Read the model definition and answer for the solid it produces. Units are mm, in the model's axes. A direction names the side the tool comes from. Coordinates: 2 decimals unless noted, no trailing zeros. Write each loop counter-clockwise with the first axis right and the second up, starting at its lowest first coordinate (ties: lowest second). Pieces come first, ordered by that corner, then holes.
from build123d import *

# Parameters (mm, degrees)
PAD002_DEPTH    = 2
FILLET003_R     = 0.4
POCKET010_DEPTH = 0.1


with BuildPart() as part:
    # Sketch009 → Pad002 (new body)
    with BuildSketch(Plane.XY):
        Polygon((-1.675, -0.66), (1.675, -0.66), (1.675, -1.66), (0.5, -1.66), (0.5, -20.32), (1.5, -20.32), (1.5, -21.82), (-1.5, -21.82), (-1.5, -20.32), (-0.5, -20.32), (-0.5, -1.66), (-1.675, -1.66), align=None)
    extrude(amount=PAD002_DEPTH)

    # Fillet003
    fillet003_edges = [part.edges().sort_by_distance(p)[0] for p in [
        (-1.675, -1.66, 1),
        (-1.675, -0.66, 1),
        (1.675, -0.66, 1),
        (1.675, -1.66, 1),
        (0.5, -1.66, 1),
        (-0.5, -1.66, 1),
        (-0.5, -20.32, 1),
        (-1.5, -20.32, 1),
        (-1.5, -21.82, 1),
        (1.5, -21.82, 1),
        (1.5, -20.32, 1),
        (0.5, -20.32, 1),
    ]]
    fillet(fillet003_edges, radius=FILLET003_R)

    # Fillet003 Face5 → Pocket010 (cut)
    with BuildSketch(Plane(origin=(0, -11.4600006044, 2), x_dir=(0, 1, 0), z_dir=(0, 0, 1))):
        with BuildLine():
            Line((9.8000006044, 1.275), (9.8000006044, 0.9))
            ThreePointArc((9.8000006044, 0.9), (9.6828433168, 0.6171572875), (9.4000006044, 0.5))
            Line((9.4000006044, 0.5), (-8.4599993956, 0.5))
            ThreePointArc((-8.4599993956, 0.5), (-8.7428421081, 0.6171572875), (-8.8599993956, 0.9))
            Line((-8.8599993956, 0.9), (-8.8599993956, 1.1))
            ThreePointArc((-8.8599993956, 1.1), (-8.9771566832, 1.3828427125), (-9.2599993956, 1.5))
            Line((-9.2599993956, 1.5), (-9.9599993956, 1.5))
            ThreePointArc((-9.9599993956, 1.5), (-10.2428421081, 1.3828427125), (-10.3599993956, 1.1))
            Line((-10.3599993956, 1.1), (-10.3599993956, -1.1))
            ThreePointArc((-10.3599993956, -1.1), (-10.2428421081, -1.3828427125), (-9.9599993956, -1.5))
            Line((-9.9599993956, -1.5), (-9.2599993956, -1.5))
            ThreePointArc((-9.2599993956, -1.5), (-8.9771566832, -1.3828427125), (-8.8599993956, -1.1))
            Line((-8.8599993956, -1.1), (-8.8599993956, -0.9))
            ThreePointArc((-8.8599993956, -0.9), (-8.7428421081, -0.6171572875), (-8.4599993956, -0.5))
            Line((-8.4599993956, -0.5), (9.4000006044, -0.5))
            ThreePointArc((9.4000006044, -0.5), (9.6828433168, -0.6171572875), (9.8000006044, -0.9))
            Line((9.8000006044, -0.9), (9.8000006044, -1.275))
            ThreePointArc((9.8000006044, -1.275), (9.9171578919, -1.5578427125), (10.2000006044, -1.675))
            Line((10.2000006044, -1.675), (10.4000006044, -1.675))
            ThreePointArc((10.4000006044, -1.675), (10.6828433168, -1.5578427125), (10.8000006044, -1.275))
            Line((10.8000006044, -1.275), (10.8000006044, 1.275))
            ThreePointArc((10.8000006044, 1.275), (10.6828433168, 1.5578427125), (10.4000006044, 1.675))
            Line((10.4000006044, 1.675), (10.2000006044, 1.675))
            ThreePointArc((10.2000006044, 1.675), (9.9171578919, 1.5578427125), (9.8000006044, 1.275))
        make_face()
    extrude(amount=-POCKET010_DEPTH, mode=Mode.SUBTRACT)


with BuildPart() as part_1:
    # Body002 placement: moved
    add(part.part.moved(Location((0, 0, 3))))


solid = part_1.part
Item 1: The part is cut by section A-A (z = 4.7). Give the vertices of the cut face in (x, y) (3 decimals), and give its area (3 significant figures).
Item 2: Given pin 1 (1 mm diameter, centred on y = -4, z = 3.5, fed in from -X); pin 2 (0.8 mm diameter, centred on y = -21, z = 4.5, fed in from +X), each flat-ended and moving along its own axis, determine where each tip first touches the part or whether it passes through.
Item 3: For faces 1 (the flat face through (0, -14, 4.9)), 2 (the flat face through (-0.5, -11, 4)), determine the directions among +Z, -Z, +X, -X, +Y, -Y from which every point of the face is accessible in a straight line to the end or side of a thin tool.
Item 4: Find the intervals of material crossed by probe 1 along Y at (x, z) = (0.9, 4.85); probe 2 along X at (y, z) = (-18, 4.3); probe 3 along Y at (x, z) = (1.3, 4.65), in increasing order.
Item 5: The part is cut by section B-B (x = -0.7). Give the vertices of the cut face in (y, z).
Item 6: Determine the mould class of faces 3 (the flat face through (0, -21.82, 4)), 4 (the flat face through (0.5, -11, 4)), 5 (the flat face through (0, -0.66, 4)), 6 (the flat face through (0, -11, 3)) for opening direction Y: +Y half, -Y half, draft (parallel to the pull), parting line (faces both ways), or undercut.
Item 7: The part is cut by section C-C (y = -14.75). Give the vertices of the cut face in (x, z), and give its area (3 significant figures).
Answer:
1. outline: (-1.675, -1.26) arc R0.4 ccw to (-1.275, -1.66) - (-0.9, -1.66) arc R0.4 cw to (-0.5, -2.06) - (-0.5, -19.92) arc R0.4 cw to (-0.9, -20.32) - (-1.1, -20.32) arc R0.4 ccw to (-1.5, -20.72) - (-1.5, -21.42) arc R0.4 ccw to (-1.1, -21.82) - (1.1, -21.82) arc R0.4 ccw to (1.5, -21.42) - (1.5, -20.72) arc R0.4 ccw to (1.1, -20.32) - (0.9, -20.32) arc R0.4 cw to (0.5, -19.92) - (0.5, -2.06) arc R0.4 cw to (0.9, -1.66) - (1.275, -1.66) arc R0.4 ccw to (1.675, -1.26) - (1.675, -1.06) arc R0.4 ccw to (1.275, -0.66) - (-1.275, -0.66) arc R0.4 ccw to (-1.675, -1.06) - close
1. area: 26.4 mm2
2. pin 1: stops at x = -0.5
2. pin 2: stops at x = 1.5
3. face 1: +Z, +X, -X, +Y, -Y
3. face 2: +Z, -Z, -X
4. probe 1: y = -21.82 to -20.32, -1.66 to -0.66
4. probe 2: x = -0.5 to 0.5
4. probe 3: y = -21.77 to -20.37, -1.66 to -0.66
5. outline: (-21.82, 3) - (-20.27, 3) - (-20.27, 4.9) - (-21.82, 4.9) - close; (-1.71, 3) - (-0.66, 3) - (-0.66, 4.9) - (-1.71, 4.9) - close
6. face 3: -Y half
6. face 4: undercut
6. face 5: +Y half
6. face 6: draft
7. outline: (-0.5, 3) - (0.5, 3) - (0.5, 4.9) - (-0.5, 4.9) - close
7. area: 1.90 mm2
